Geometry check sheet. Reference: the model listing, model coordinates, mm. Give positions to 0.01 mm unless a question says otherwise; leave off trailing zeros. Loops run counter-clockwise (first coordinate to the right, second up) from the corner with the lowest first, then second, coordinate; pieces in that order, holes last.
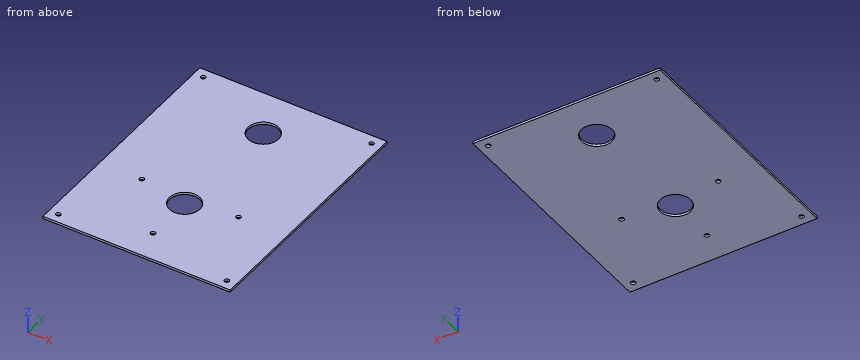
```python
from build123d import *

# Parameters (mm, degrees)
SKETCH1_W           = 254
SKETCH1_H           = 330.2
BOSS_EXTRUDE1_DEPTH = 3.175
SKETCH2_R           = 20.701
CUT_EXTRUDE1_DEPTH  = 301.262663605
SKETCH3_R           = 3.3
SKETCH3_R_2         = 20.6375
SKETCH3_R_3         = 3.2512
CUT_EXTRUDE2_DEPTH  = 301.262663605


with BuildPart() as part:
    # Sketch1 → Boss-Extrude1 (new body)
    with BuildSketch(Plane.XY):
        with Locations((19.981406387, -96.70919141)):
            Rectangle(SKETCH1_W, SKETCH1_H)
    extrude(amount=-BOSS_EXTRUDE1_DEPTH)

    # Sketch2 → Cut-Extrude1 (cut, through all)
    with BuildSketch(Plane.XY):
        with Locations((19.981406387, 4.89080859)):
            Circle(SKETCH2_R)
    extrude(amount=-CUT_EXTRUDE1_DEPTH, mode=Mode.SUBTRACT)

    # Sketch3 → Cut-Extrude2 (cut, through all)
    with BuildSketch(Plane.XY):
        with Locations((-50.007395692, -142.229557515)):
            Circle(SKETCH3_R)
        with Locations((81.218237397, -142.229557515)):
            Circle(SKETCH3_R)
        with Locations((15.605420852, -220.423867352)):
            Circle(SKETCH3_R)
        with Locations((15.605420852, -153.798867352)):
            Circle(SKETCH3_R_2)
        with Locations((134.281406387, 55.69080859)):
            Circle(SKETCH3_R_3)
        with Locations((-94.318593613, 55.69080859)):
            Circle(SKETCH3_R_3)
        with Locations((134.281406387, -249.10919141)):
            Circle(SKETCH3_R_3)
        with Locations((-94.318593613, -249.10919141)):
            Circle(SKETCH3_R_3)
    extrude(amount=-CUT_EXTRUDE2_DEPTH, mode=Mode.SUBTRACT)


solid = part.part
```
1) Sectioned sample at B-B on z = -2.5. Count the separate pieces of the cut face and the enclosed holes in it, plus the area to 3 significant figures.
2) Sectioned sample at A-A on x = 25. Enter the section's corners in (y, z) (3 decimals), plus the area to 3 significant figures.
3) Scan lines: line 1 along Y through (x, z) = (-94, -0.25); line 2 along X through (y, z) = (-248, -1.8); line 3 along X through (y, z) = (-153, -1.4). Record each from-to range of solid material in increasing order.
4) Depth check by flat-ended pin: P1, Ø6, axis at x = 134.28, y = 55.69, coming from the -Z side. Enter the tip coordinate at first touch or a pass-through.
Determined:
1. separate pieces: 1
1. enclosed holes: 9
1. area: 81,000 mm2
2. outline: (-261.809, -3.175) - (-172.174, -3.175) - (-172.174, 0) - (-261.809, 0) - close; (-135.424, -3.175) - (-15.193, -3.175) - (-15.193, 0) - (-135.424, 0) - close; (24.974, -3.175) - (68.391, -3.175) - (68.391, 0) - (24.974, 0) - close
2. area: 804 mm2
3. line 1: y = -261.81 to -252.34, -245.87 to 52.46, 58.93 to 68.39
3. line 2: x = -107.02 to -97.37, -91.26 to 131.23, 137.34 to 146.98
3. line 3: x = -107.02 to -5.02, 36.23 to 146.98
4. P1: passes through
